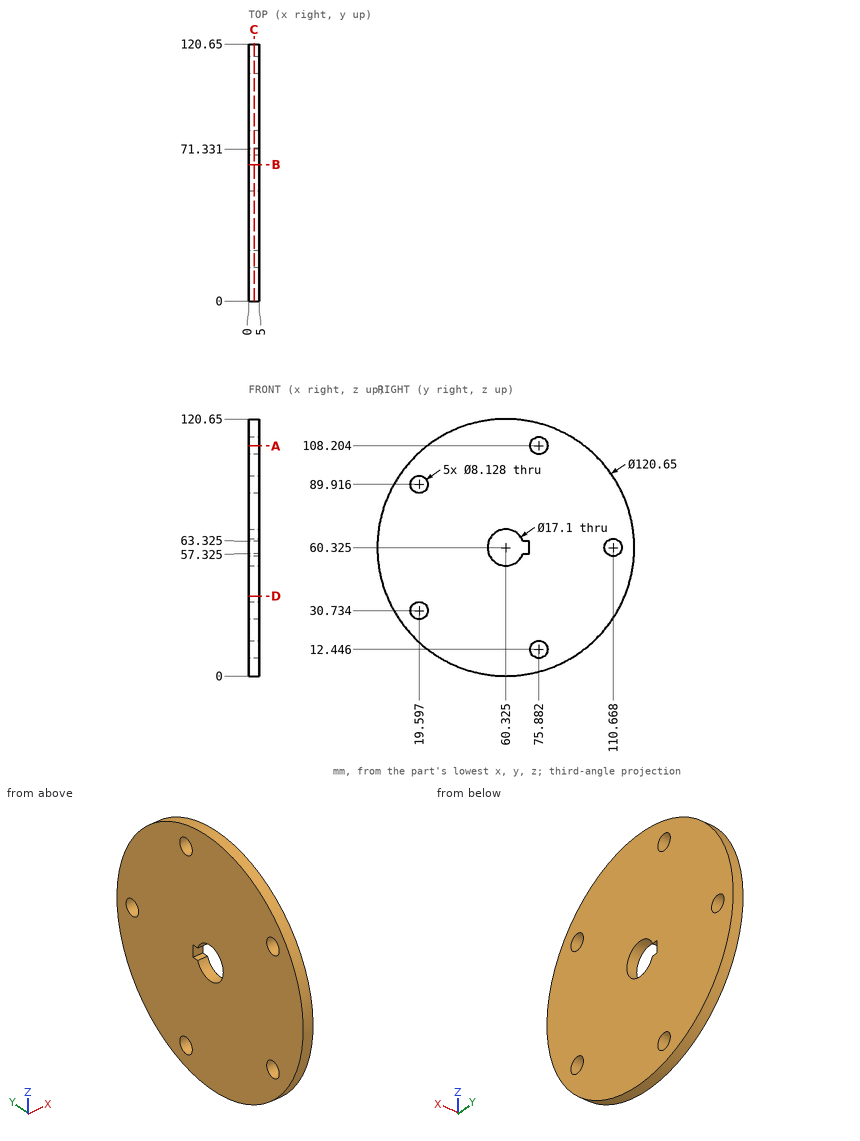
Answer from the drawing. Dimensions are ordinates in mm from the lowest x, y and z of the part. Coordinates: 2 decimals unless noted, no trailing zeros. Write each loop counter-clockwise with the first axis right and the second up, starting at its lowest first coordinate (ties: lowest second). Pieces come first, ordered by that corner, then holes. Notation, with made-up numbers: (65, -28) - (123, -28) arc R35 cw to (123, 8) - close; hole circle Ø1 at (-18.75, 50). An arc over 180 degrees is marked (long way). Return JSON: item names as keys, results as strings. Group by question number.
Q1. The part is cut by section B-B on y = 64. Write down the section's boundary in (x, z) (1 decimal), and give its area (3 significant figures).
Q2. Flat-ended cylindrical pins translate along their axes: pin 1 Ø1 at (x, y) = (2, 95.5) entering from -Z; pin 2 Ø2 at (x, y) = (1, 69.5) entering from -Z; pin 3 Ø1.5 at (x, y) = (2.5, 69.5) entering from +Z. Find the tip coordinate at first contact, or state that the pin passes through.
Q3. The part is cut by section A-A on z = 108. Write down the section's boundary in (x, y).
Q4. Find the intervals of material crossed by line 1 along Y through (x, z) = (3.85, 63) (1 decimal); line 2 along Y through (x, z) = (4.3, 59) (1 decimal); line 3 along Z through (x, y) = (1.25, 37), in increasing order. Write a range as [from, to].
Q5. The part is cut by section D-D on z = 37.5. Write down the section's boundary in (x, y) (1 decimal).
Q6. The part is cut by section C-C on x = 2.6. State how many separate pieces and enclosed holes the cut face has, and give its area (3 significant figures).
Evaluation:
{
 "1": {"outline": "(0, 0.1) - (5, 0.1) - (5, 52.6) - (0, 52.6) - close; (0, 68) - (5, 68) - (5, 120.5) - (0, 120.5) - close", "area": "525 mm2"},
 "2": {"pin 1": "stops at z = 10.96", "pin 2": "stops at z = 0.56", "pin 3": "stops at z = 120.06"},
 "3": {"outline": "(0, 23.36) - (5, 23.36) - (5, 71.82) - (0, 71.82) - close; (0, 79.94) - (5, 79.94) - (5, 97.29) - (0, 97.29) - close"},
 "4": {"line 1": "y = [0.1, 52.2], [71.3, 107.6], [113.7, 120.6]", "line 2": "y = [0, 51.9], [71.3, 106.8], [114.5, 120.6]", "line 3": "z = [4.69, 115.96]"},
 "5": {"outline": "(0, 4.5) - (5, 4.5) - (5, 116.2) - (0, 116.2) - close"},
 "6": {"separate pieces": "1", "enclosed holes": "6", "area": "10,900 mm2"}
}
